Check sheet for the modelled part. Datum: model origin and axes. Units: mm. A direction names the side the tool comes from. Give positions to 0.01 mm unless a question says otherwise; leave off trailing zeros. Write each loop counter-clockwise with the first axis right and the second up, starting at its lowest first coordinate (ties: lowest second). Pieces come first, ordered by that corner, then holes. Notation, with made-up numbers: (41.5, 72.5) -> (64.5, 72.5) arc R21 cw to (64.5, 93.5) -> close; hole circle Ø5 at (-22, -8.75). An arc over 180 degrees is marked (long way). Return JSON: item names as keys, results as strings.
from build123d import *

# Parameters (mm, degrees)
SKETCH_1_W                         = 2
SKETCH_1_H                         = 500
SM_BASE_FLANGE_1_DEPTH             = 220
SM_EDGE_FLANGE_1_STRIP_W           = 11.6
SM_EDGE_FLANGE_1_STRIP_H           = 2
SM_EDGE_FLANGE_1_STRIP_CUT_DEPTH   = 500
SM_EDGE_FLANGE_1_STRIP_2_W         = 11.6
SM_EDGE_FLANGE_1_STRIP_2_H         = 2
SM_EDGE_FLANGE_1_STRIP_CUT_2_DEPTH = 500
SM_EDGE_FLANGE_1_DEPTH             = 500
SM_EDGE_FLANGE_1_BEND_DEPTH        = 500
SKETCH_10_W                        = 3
SKETCH_10_H                        = 50
CUT_EXTRUDE_1_DEPTH                = 550.545266561
HOLE_WIZARD_M81_D                  = 9
HOLE_WIZARD_M81_DEPTH              = 5
HOLE_WIZARD_M81_TIP                = 2.703872786
HOLE_WIZARD_M61_D                  = 6.6


# Sheet-metal steps are written as plain solids
with BuildPart() as part:
    # Sketch 1 → Базовая кромка1 (new body)
    with BuildSketch(Plane.XY):
        with Locations((1, 250)):
            Rectangle(SKETCH_1_W, SKETCH_1_H)
    extrude(amount=SM_BASE_FLANGE_1_DEPTH)

    # Ребро-кромка1 strip (across the edge) → Ребро-кромка1 strip cut (cut)
    with BuildSketch(Plane(origin=(2, 0, 0), x_dir=(0, 0, 1), z_dir=(0, 1, 0))):
        with Locations((-2, -1)):
            Rectangle(SM_EDGE_FLANGE_1_STRIP_W, SM_EDGE_FLANGE_1_STRIP_H)
    extrude(amount=SM_EDGE_FLANGE_1_STRIP_CUT_DEPTH, mode=Mode.SUBTRACT)

    # Ребро-кромка1 strip 2 (across the edge) → Ребро-кромка1 strip cut 2 (cut)
    with BuildSketch(Plane(origin=(2, 500, 220), x_dir=(0, 0, -1), z_dir=(0, -1, 0))):
        with Locations((-2, -1)):
            Rectangle(SM_EDGE_FLANGE_1_STRIP_2_W, SM_EDGE_FLANGE_1_STRIP_2_H)
    extrude(amount=SM_EDGE_FLANGE_1_STRIP_CUT_2_DEPTH, mode=Mode.SUBTRACT)

    # Ребро-кромка1 section (across the edge) → Ребро-кромка1 (add)
    with BuildSketch(Plane(origin=(2, 0, 0), x_dir=(0, 0, 1), z_dir=(0, 1, 0))):
        with BuildLine():
            Line((0, 1.8), (0, 58))
            Line((0, 58), (2, 58))
            Line((2, 58), (2, 1.8))
            ThreePointArc((2, 1.8), (2.527207794, 0.527207794), (3.8, 0))
            Line((3.8, 0), (3.8, -2))
            ThreePointArc((3.8, -2), (1.112994231, -0.887005769), (0, 1.8))
        make_face()
    extrude(amount=SM_EDGE_FLANGE_1_DEPTH)

    # Ребро-кромка1 section 2 (across the edge) → Ребро-кромка1 bend (add)
    with BuildSketch(Plane(origin=(2, 500, 220), x_dir=(0, 0, -1), z_dir=(0, -1, 0))):
        with BuildLine():
            Line((0, 1.8), (0, 58))
            Line((0, 58), (2, 58))
            Line((2, 58), (2, 1.8))
            ThreePointArc((2, 1.8), (2.527207794, 0.527207794), (3.8, 0))
            Line((3.8, 0), (3.8, -2))
            ThreePointArc((3.8, -2), (1.112994231, -0.887005769), (0, 1.8))
        make_face()
    extrude(amount=SM_EDGE_FLANGE_1_BEND_DEPTH)

    # Эскиз10 → Вырез-Вытянуть1 (cut, through all)
    with BuildSketch(Plane(origin=(0, 0, 0), x_dir=(-1, 0, 0), z_dir=(0, 0, -1))):
        with Locations((-58.5, 25)):
            Rectangle(SKETCH_10_W, SKETCH_10_H)
    extrude(amount=-CUT_EXTRUDE_1_DEPTH, mode=Mode.SUBTRACT)

    # Отверстие с зазором M81
    with Locations(Plane(origin=(2, 0, 0), x_dir=(0, 0, -1), z_dir=(1, 0, 0))):
        with Locations((-30, 25), (-110, 25), (-190, 25)):
            Hole(HOLE_WIZARD_M81_D / 2, depth=HOLE_WIZARD_M81_DEPTH)
            with Locations((0, 0, -(HOLE_WIZARD_M81_DEPTH + HOLE_WIZARD_M81_TIP / 2))):  # 118° drill point
                Cone(0, HOLE_WIZARD_M81_D / 2, HOLE_WIZARD_M81_TIP, mode=Mode.SUBTRACT)

    # Отверстие с зазором M61 (through all)
    with Locations(Plane(origin=(0, 0, 0), x_dir=(-1, 0, 0), z_dir=(0, 0, -1))):
        with Locations((-20, 475), (-20, 425), (-20, 375), (-20, 325), (-20, 275), (-20, 225), (-20, 175), (-20, 125), (-20, 75)):
            Hole(HOLE_WIZARD_M61_D / 2)


solid = part.part
(1) Cross-section at B-B on x = 10.5. Enter the section's corners in (y, z), then the cut area to 3 significant figures.
Reply:
{"outline": "(0, 0) -> (500, 0) -> (500, 2) -> (0, 2) -> close; (0, 218) -> (500, 218) -> (500, 220) -> (0, 220) -> close", "area": "2,000 mm^2"}
(2) Thickness scan on L1, parallel to Z at x = 45.5, y = 399.5; L2, parallel to X at y = 240, z = 20; L3, parallel to X at y = 275, z = 1.55. Record the ranges inside material, lowest first.
Reply:
{"L1": "0 to 2, 218 to 220", "L2": "0 to 2", "L3": "0.74 to 16.7, 23.3 to 60"}
(3) Set-up check for faces 4 (the flat face through (2, 247, 109)), 5 (the flat face through (32, 254, 220)): record each of +Z, -Z, +X, -X, +Y, -Y from which the full face is reachable in a straight line by a thin tool's end or side.
Reply:
{"face 4": "+X, +Y, -Y", "face 5": "+Z, +X, -X, +Y, -Y"}
(4) Depth check by flat-ended pin: pin 1 Ø12 at (x, y) = (43, 444.5) entering from -Z; pin 2 Ø12 at (y, z) = (301, 177) entering from +X; pin 3 Ø0.6 at (y, z) = (28.5, 1) entering from +X. Enter the tip coordinate at first touch or a pass-through.
Reply:
{"pin 1": "z = 0", "pin 2": "x = 2", "pin 3": "x = 57"}
(5) Cross-section at A-A on z = 190. Enter the section's corners in (x, y), then the cut area to 3 significant figures.
Reply:
{"outline": "(0, 0) -> (2, 0) -> (2, 20.5) -> (0, 20.5) -> close; (0, 29.5) -> (2, 29.5) -> (2, 500) -> (0, 500) -> close", "area": "982 mm^2"}
(6) Release check for a two-part mould opening along Z. For faces 1 (the cylindrical face through (0.986, 28.794, 32.419)), 2 (the flat face through (32, 246, 0)), 3 (the flat face through (1, 500, 109)) record: pulls with the +Z half, pulls with the -Z half, needs draft (parallel to the pull), parting line crosses it, or undercut.
Reply:
{"face 1": "undercut", "face 2": "pulls with the -Z half", "face 3": "needs draft"}
(7) Cross-section at C-C on y = 101. Enter the section's corners in (x, z).
Reply:
{"outline": "(0, 3.8) arc R3.8 ccw to (3.8, 0) -> (60, 0) -> (60, 2) -> (3.8, 2) arc R1.8 cw to (2, 3.8) -> (2, 216.2) arc R1.8 cw to (3.8, 218) -> (60, 218) -> (60, 220) -> (3.8, 220) arc R3.8 ccw to (0, 216.2) -> close"}
